Read the model definition and answer for the solid it produces. Units are mm, in the model's axes. Face numbers are marked on the shaded views. A direction names the side the tool comes from. Coordinates: 2 decimals unless noted, no trailing zeros. Write each loop counter-clockwise with the first axis right and the second up, starting at its lowest first coordinate (ties: lowest second). Pieces come first, ordered by that corner, then holes. Notation, with made-up numbers: (-18.75, 65.25) -> (32.25, 65.25) arc R26 cw to (32.25, 82.25) -> close; hole circle Ø7 at (77.5, -9). An arc over 180 degrees is marked (long way). Answer in a Markdown table with one row per item. Add a question column.
Item 1: Section B-B on z = 19.75 is taken. Write down the section's boundary in (x, y).
Item 2: Straight lines are drawn through the part: line 1 (Y direction, x = 0, z = 19.5); line 2 (Y direction, x = -0.25, z = 6) (3 decimals); line 3 (Z direction, x = -4.25, y = 2). For each, find the intervals that lie inside material, in ascending order. Write a range as from..to.
Item 3: Section A-A on x = 0 is taken. Write down the section's boundary in (y, z) (3 decimals).
Item 4: Given pin 1 Ø1.1 at (x, y) = (1, 0.5) entering from -Z; pin 2 Ø3 at (x, z) = (1, 14) entering from +Y; pin 3 Ø3 at (x, z) = (-3, 18) entering from -Y, each flat-ended and moving along its own axis, determine where each tip first touches the part or whether it passes through.
Item 5: For a pull along Y with two mould halves and no side action, classify the marked faces 5, 6 and 7 as +Y half, -Y half, draft (parallel to the pull), parting line (faces both ways), or undercut.
Item 6: Which of the six approach directions +Z, -Z, +X, -X, +Y, -Y give full straight-line access (tool end or side, diameter ignored) to the marked faces 1, 2, 3 and 4?
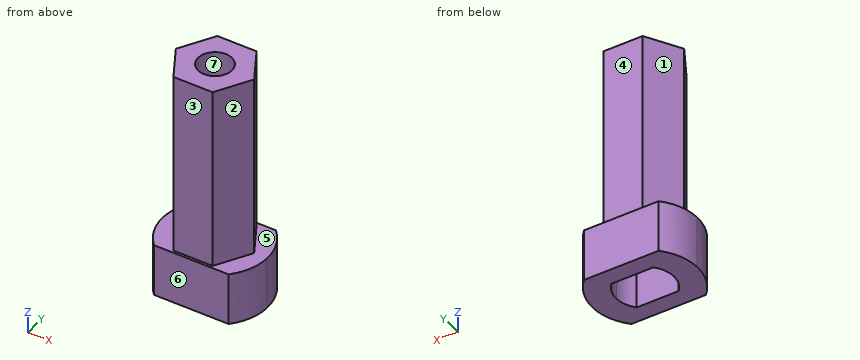
```python
from build123d import *

# Parameters (mm, degrees)
EXTRUDE_1_DEPTH     = 5
EXTRUDE_2_DEPTH     = 17.5
SKETCH_3_R          = 1.6
CUT_EXTRUDE_1_DEPTH = 24.313086454
CUT_EXTRUDE_START   = -8
CUT_EXTRUDE_2_DEPTH = 8


with BuildPart() as part:
    # 草图1 → 凸台-拉伸1 (new body)
    with BuildSketch(Plane.XY):
        with BuildLine():
            ThreePointArc((-3.570714214, 3.5), (-4.628907596, 1.890294809), (-5, 0))
            Line((-5, 0), (5, 0))
            ThreePointArc((5, 0), (4.628907596, 1.890294809), (3.570714214, 3.5))
            Line((3.570714214, 3.5), (-3.570714214, 3.5))
        make_face()
        with BuildLine():
            Line((5, 0), (-5, 0))
            ThreePointArc((-5, 0), (-4.628907596, -1.890294809), (-3.570714214, -3.5))
            Line((-3.570714214, -3.5), (3.570714214, -3.5))
            ThreePointArc((3.570714214, -3.5), (4.628907596, -1.890294809), (5, 0))
        make_face()
    extrude(amount=EXTRUDE_1_DEPTH)

    # 草图2 → 凸台-拉伸2 (add)
    with BuildSketch(Plane.XY.offset(5)):
        Polygon((1.876388375, 3.25), (-1.876388375, 3.25), (-3.75277675, 0), (-1.876388375, -3.25), (1.876388375, -3.25), (3.75277675, 0), align=None)
    extrude(amount=EXTRUDE_2_DEPTH)

    # 草图3 → 切除-拉伸1 (cut, through all)
    with BuildSketch(Plane.XY.offset(22.5)):
        Circle(SKETCH_3_R)
    extrude(amount=-CUT_EXTRUDE_1_DEPTH, mode=Mode.SUBTRACT)

    # 草图4 → 切除-拉伸2 (cut)
    with BuildSketch(Plane(origin=(0, 0, 0), x_dir=(-1, 0, 0), z_dir=(0, 0, -1)).offset(CUT_EXTRUDE_START)):
        with BuildLine():
            Line((2.011684617, 1.875), (-2.011684617, 1.875))
            ThreePointArc((-2.011684617, 1.875), (-2.55877243, 1.007563224), (-2.75, 0))
            Line((-2.75, 0), (-1.6, 0))
            ThreePointArc((-1.6, 0), (0, 1.6), (1.6, 0))
            Line((1.6, 0), (2.75, 0))
            ThreePointArc((2.75, 0), (2.55877243, 1.007563224), (2.011684617, 1.875))
        make_face()
        with BuildLine():
            Line((-1.6, 0), (-2.75, 0))
            ThreePointArc((-2.75, 0), (-2.55877243, -1.007563224), (-2.011684617, -1.875))
            Line((-2.011684617, -1.875), (2.011684617, -1.875))
            ThreePointArc((2.011684617, -1.875), (2.55877243, -1.007563224), (2.75, 0))
            Line((2.75, 0), (1.6, 0))
            ThreePointArc((1.6, 0), (0, -1.6), (-1.6, 0))
        make_face()
    extrude(amount=CUT_EXTRUDE_2_DEPTH, mode=Mode.SUBTRACT)


solid = part.part
```
Results below:
| question | item | result |
|---|---|---|
| 1 | outline | (-3.75, 0) -> (-1.88, -3.25) -> (1.88, -3.25) -> (3.75, 0) -> (1.88, 3.25) -> (-1.88, 3.25) -> close; hole circle Ø3.2 at (0, 0) |
| 2 | line 1 | y = -3.25..-1.6, 1.6..3.25 |
| 2 | line 2 | y = -3.25..-1.875, 1.875..3.25 |
| 2 | line 3 | z = 0..5 |
| 3 | outline | (-3.5, 0) -> (-1.875, 0) -> (-1.875, 8) -> (-1.6, 8) -> (-1.6, 22.5) -> (-3.25, 22.5) -> (-3.25, 5) -> (-3.5, 5) -> close; (1.6, 8) -> (1.875, 8) -> (1.875, 0) -> (3.5, 0) -> (3.5, 5) -> (3.25, 5) -> (3.25, 22.5) -> (1.6, 22.5) -> close |
| 4 | pin 1 | stops at z = 8 |
| 4 | pin 2 | stops at y = 3.25 |
| 4 | pin 3 | stops at y = -3.25 |
| 5 | face 5 | draft |
| 5 | face 6 | -Y half |
| 5 | face 7 | undercut |
| 6 | face 1 | +Z, -X, +Y |
| 6 | face 2 | +Z, +X, -Y |
| 6 | face 3 | +Z, +X, -X, -Y |
| 6 | face 4 | +Z, +X, -X, +Y |
